Geometry check sheet. Reference: the model listing, model coordinates, mm. Face numbers are marked on the shaded views. A direction names the side the tool comes from. Give positions to 0.01 mm unless a question says otherwise; leave off trailing zeros. Write each loop counter-clockwise with the first axis right and the second up, starting at its lowest first coordinate (ties: lowest second). Pieces come first, ordered by that corner, then holes. Notation, with made-up numbers: M -36.5,68 L -26.5,68 A25 cw -26.5,94 Z; hole C 48,22 d11. An arc over 180 degrees is marked long. One line per item, written item: value. Start each with the question number.
1. Scan lines: line 1 (X direction, y = 31, z = 146.5); line 2 (Z direction, x = 209.55, y = -92); line 3 (Z direction, x = -266, y = 74). Record each from-to range of solid material in increasing order.
2. Tool access check on the marked faces 1, 2, 3, 4 and 5. Record the directions out of +Z, -Z, +X, -X, +Y, -Y that give a thin tool (end or side, any length) a straight path to the whole face; none if there is none.
3. Cross-section at B-B on y = -54. Record the cut outline in (x, z).
4. Gauge pin test, flat end, axial feed: pin 1 (20.5 mm diameter, centred on x = 209.55, z = 152.4, fed in from -Y). Record the tip position at first contact, or that the pin passes through.
5. Cross-section at A-A on x = -209.55. Record the cut outline in (y, z).
6. Release check for a two-part mould opening along Z. For the marked faces 6, 7, 8 and 9 record: pulls with the +Z half, pulls with the -Z half, needs draft (parallel to the pull), parting line crosses it, or undercut.
7. Cross-section at C-C on z = 243.5. Record the cut outline in (x, y).
8. Cross-section at D-D on x = 0. Record the cut outline in (y, z).
from build123d import *
from build123d import SkipClean  # not in build123d's __all__

# Parameters (mm, degrees)
F0_W      = 203.2
F0_H      = 203.2
F1_DEPTH  = 12.7
F2_W      = 203.2
F2_H      = 203.2
F2_W_2    = 177.8
F2_H_2    = 177.8
F3_DEPTH  = 254
F4_W      = 203.2
F4_H      = 203.2
F4_W_2    = 177.8
F4_H_2    = 177.8
F5_DEPTH  = 12.7
F6_W      = 203.2
F6_H      = 203.2
F7_DEPTH  = 12.7
F8_W      = 203.2
F8_H      = 203.2
F8_W_2    = 177.8
F8_H_2    = 177.8
F9_DEPTH  = 203.2
F10_W     = 12.7
F10_H     = 177.8
F11_DEPTH = 177.8
F12_R     = 50.8
F12_R_2   = 12.7
F12_R_3   = 82.55
F13_DEPTH = 25.4
F15_DEPTH = 203.2


with BuildPart() as f1:
    # F0 (on Top) → F1 (new body)
    with BuildSketch(Plane.XY):
        Rectangle(F0_W, F0_H)
    extrude(amount=F1_DEPTH)

    # F2 (on face) → F3 (join)
    with BuildSketch(Plane.XY.offset(12.7)):
        Rectangle(F2_W, F2_H)
        Rectangle(F2_W_2, F2_H_2, mode=Mode.SUBTRACT)
    extrude(amount=F3_DEPTH)

    # F4 (on face) → F5 (join)
    with BuildSketch(Plane.XY.offset(266.7)):
        Rectangle(F4_W, F4_H)
        Rectangle(F4_W_2, F4_H_2, mode=Mode.SUBTRACT)
        Rectangle(F4_W_2, F4_H_2)
    extrude(amount=-F5_DEPTH)

    # F6 (on face) → F7 (join)
    with BuildSketch(Plane(origin=(-101.6, 0, 0), x_dir=(0, -1, 0), z_dir=(-1, 0, 0))):
        with Locations((0, 101.6)):
            Rectangle(F6_W, F6_H)
    extrude(amount=F7_DEPTH)

    # F8 (on face) → F9 (join)
    with BuildSketch(Plane(origin=(-114.3, 0, 0), x_dir=(0, -1, 0), z_dir=(-1, 0, 0))):
        with Locations((0, 101.6)):
            Rectangle(F8_W, F8_H)
        with Locations((0, 101.6)):
            Rectangle(F8_W_2, F8_H_2, mode=Mode.SUBTRACT)
    extrude(amount=F9_DEPTH)

    # F10 (on face) → F11 (join)
    with BuildSketch(Plane.XY.offset(12.7)):
        with Locations((-311.15, 0)):
            Rectangle(F10_W, F10_H)
    extrude(amount=F11_DEPTH)

    # F12 (on face) → F13 (cut)
    with BuildSketch(Plane.XZ.offset(101.6)):
        with Locations((-209.55, 76.2)):
            Circle(F12_R)
        with Locations((-209.55, 152.4)):
            Circle(F12_R_2)
        with Locations((0, 133.35)):
            Circle(F12_R_3)
    extrude(amount=-F13_DEPTH, mode=Mode.SUBTRACT)

    # F14 (on face) → F15 (cut)
    with BuildSketch(Plane.XZ.offset(101.6)):
        with BuildLine():
            Line((101.6, 0), (101.6, 266.7))
            Line((101.6, 266.7), (0, 266.7))
            Line((0, 266.7), (0, 215.9))
            ThreePointArc((0, 215.9), (58.3716647869, 191.7216647869), (82.55, 133.35))
            ThreePointArc((82.55, 133.35), (58.3716647869, 74.9783352131), (0, 50.8))
            Line((0, 50.8), (0, 0))
            Line((0, 0), (101.6, 0))
        make_face()
        with BuildLine():
            ThreePointArc((82.55, 133.35), (58.3716647869, 191.7216647869), (0, 215.9))
            Line((0, 215.9), (0, 50.8))
            ThreePointArc((0, 50.8), (58.3716647869, 74.9783352131), (82.55, 133.35))
        make_face()
    extrude(amount=-F15_DEPTH, mode=Mode.SUBTRACT)

    # F16: F1 across face


with BuildPart() as f1_1:
    add(f1.part, clean=False)
    with SkipClean():  # cleaning this boolean's faces spoils the solid; the shape is the same uncleaned
        add(f1.part.mirror(Plane(origin=(0, 21.7236842105, 133.35), x_dir=(0, 1, 0), z_dir=(1, 0, 0))), clean=False)


solid = f1_1.part
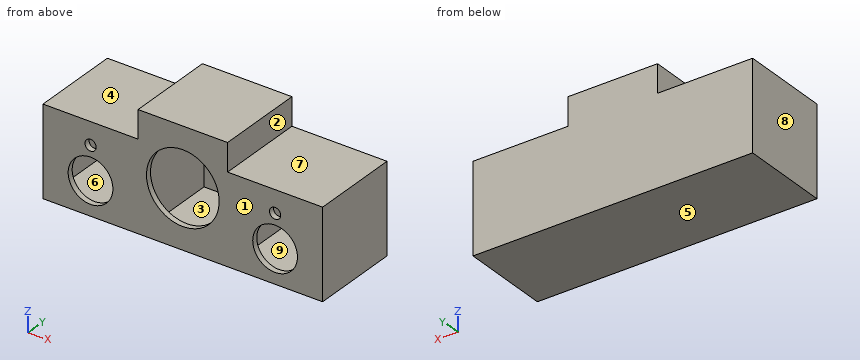
Report:
1. line 1: x = -317.5 to -304.8, -114.3 to -88.9, 88.9 to 114.3, 304.8 to 317.5
1. line 2: z = 0 to 25.4, 127 to 139.7, 165.1 to 203.2
1. line 3: z = 0 to 12.7, 190.5 to 203.2
2. face 1: +Z, -Z, +X, -X, -Y
2. face 2: +Z, +X, +Y, -Y
2. face 3: none
2. face 4: +Z, -X, +Y, -Y
2. face 5: -Z, +X, -X, +Y, -Y
3. outline: M -317.5,0 L 317.5,0 L 317.5,203.2 L 101.6,203.2 L 101.6,266.7 L -101.6,266.7 L -101.6,203.2 L -317.5,203.2 Z; hole M -304.8,12.7 L -114.3,12.7 L -114.3,190.5 L -304.8,190.5 Z; hole M -88.9,12.7 L 88.9,12.7 L 88.9,254 L -88.9,254 Z; hole M 114.3,12.7 L 304.8,12.7 L 304.8,190.5 L 114.3,190.5 Z
4. pin 1: stops at y = 88.9
5. outline: M -101.6,0 L 101.6,0 L 101.6,203.2 L -101.6,203.2 L -101.6,165.1 L -88.9,165.1 L -88.9,190.5 L 88.9,190.5 L 88.9,12.7 L -88.9,12.7 L -88.9,25.4 L -101.6,25.4 Z; M -101.6,127 L -88.9,127 L -88.9,139.7 L -101.6,139.7 Z
6. face 6: undercut
6. face 7: pulls with the +Z half
6. face 8: needs draft
6. face 9: undercut
7. outline: M -101.6,-101.6 L 101.6,-101.6 L 101.6,101.6 L -101.6,101.6 Z; hole M -88.9,-88.9 L 88.9,-88.9 L 88.9,88.9 L -88.9,88.9 Z
8. outline: M -101.6,0 L 101.6,0 L 101.6,266.7 L -101.6,266.7 L -101.6,215.9 L -88.9,215.9 L -88.9,254 L 88.9,254 L 88.9,12.7 L -88.9,12.7 L -88.9,50.8 L -101.6,50.8 Z
